Work out the finished part from the listing and answer in its coordinate system (mm). A direction names the side the tool comes from. Coordinates: 2 decimals unless noted, no trailing zeros. Order: outer loops, then holes, each group sorted by start corner. A loop starts at its lowest first (then second) coordinate and runs counter-clockwise, first axis right, second up.
```python
from build123d import *

# Parameters (mm, degrees)
BOSS_EXTRUDE1_DEPTH            = 5
FILLET1_R                      = 5
M3X0_5_TAPPED_HOLE1_AT_2_COUNT = 2
M3X0_5_TAPPED_HOLE1_AT_2_PITCH = 10
M2_5X0_45_TAPPED_HOLE2_D       = 2.05
CUT_EXTRUDE1_DEPTH             = 5
FILLET2_R                      = 3
M2_5X0_45_TAPPED_HOLE1_D       = 2.05


with BuildPart() as part:
    # Sketch1 → Boss-Extrude1 (new body)
    with BuildSketch(Plane(origin=(0, 0, 0), x_dir=(1, 0, 0), z_dir=(0, 1, 0))):
        with BuildLine():
            Line((-20.784609691, 33), (20.784609691, 33))
            ThreePointArc((20.784609691, 33), (39, 0), (20.784609691, -33))
            Line((20.784609691, -33), (-20.784609691, -33))
            ThreePointArc((-20.784609691, -33), (-39, 0), (-20.784609691, 33))
        make_face()
    extrude(amount=BOSS_EXTRUDE1_DEPTH)

    # Fillet1
    fillet1_edges = [part.edges().sort_by_distance(p)[0] for p in [
        (-20.784609691, 2.5, -33),
        (20.784609691, 2.5, -33),
        (20.784609691, 2.5, 33),
        (-20.784609691, 2.5, 33),
    ]]
    fillet(fillet1_edges, radius=FILLET1_R)

    # Sketch3 → M3x0.5 Tapped Hole1 (revolve, cut)
    with BuildSketch(Plane(origin=(-5, 2.5, 33), x_dir=(0, -1, 0), z_dir=(1, 0, 0))):
        Polygon((0, 0), (0, 8.251075774), (1.25, 7.5), (1.25, 0), align=None)
    m3x0_5_tapped_hole1 = revolve(axis=Axis((-5, 2.5, 39.35), (0, 0, -1)), mode=Mode.SUBTRACT)

    # M3x0.5 Tapped Hole1 at 2: M3x0.5 Tapped Hole1 ×2
    with Locations(*[(i * M3X0_5_TAPPED_HOLE1_AT_2_PITCH, 0, 0) for i in range(1, M3X0_5_TAPPED_HOLE1_AT_2_COUNT)]):
        add(m3x0_5_tapped_hole1, mode=Mode.SUBTRACT)

    # Mirror1: M3x0.5 Tapped Hole1 across plane
    add(m3x0_5_tapped_hole1.mirror(Plane.XY), mode=Mode.SUBTRACT)

    # Mirror1 copy 1 sketch → Mirror1 copy 1 (revolve, cut)
    with BuildSketch(Plane(origin=(5, 2.5, -33), x_dir=(0, -1, 0), z_dir=(1, 0, 0))):
        Polygon((0, 0), (0, -8.251075774), (1.25, -7.5), (1.25, 0), align=None)
    revolve(axis=Axis((5, 2.5, -39.35), (0, 0, -1)), mode=Mode.SUBTRACT)

    # M2.5x0.45 Tapped Hole2 (through all)
    with Locations(Plane(origin=(0, 0, 0), x_dir=(-1, 0, 0), z_dir=(0, -1, 0))):
        with Locations((12.5, -5), (-12.5, -5), (0, 3)):
            Hole(M2_5X0_45_TAPPED_HOLE2_D / 2)

    # Sketch6 → Cut-Extrude1 (cut)
    with BuildSketch(Plane.XZ):
        with BuildLine():
            Line((-31.749015733, 9), (31.749015733, 9))
            ThreePointArc((31.749015733, 9), (26.910919894, 19.099800796), (18.973665961, 27))
            Line((18.973665961, 27), (-18.973665961, 27))
            ThreePointArc((-18.973665961, 27), (-26.910919894, 19.099800796), (-31.749015733, 9))
        make_face()
        with BuildLine():
            Line((32.984845005, 1), (10.5, 1))
            Line((10.5, 1), (2.5, -7))
            Line((2.5, -7), (-2.5, -7))
            Line((-2.5, -7), (-10.5, 1))
            Line((-10.5, 1), (-32.984845005, 1))
            ThreePointArc((-32.984845005, 1), (-29.511382812, -14.767473872), (-18.973665961, -27))
            Line((-18.973665961, -27), (18.973665961, -27))
            ThreePointArc((18.973665961, -27), (29.511382812, -14.767473872), (32.984845005, 1))
        make_face()
    extrude(amount=-CUT_EXTRUDE1_DEPTH, mode=Mode.SUBTRACT)

    # Fillet2
    fillet2_edges = [part.edges().sort_by_distance(p)[0] for p in [
        (10.5, 2.5, 1),
        (2.5, 2.5, -7),
        (-2.5, 2.5, -7),
        (-10.5, 2.5, 1),
        (-32.984845005, 2.5, 1),
        (-18.973665961, 2.5, -27),
        (32.984845005, 2.5, 1),
        (-18.973665961, 2.5, 27),
        (31.749015733, 2.5, 9),
        (18.973665961, 2.5, 27),
        (-31.749015733, 2.5, 9),
        (18.973665961, 2.5, -27),
    ]]
    fillet(fillet2_edges, radius=FILLET2_R)

    # M2.5x0.45 Tapped Hole1 (through all)
    with Locations(Plane(origin=(0, 0, 0), x_dir=(-1, 0, 0), z_dir=(0, -1, 0))):
        with Locations((-21.15, -28.5), (21.15, -28.5), (30.3, 18.5), (-30.3, 18.5), (-35.15, -5), (35.15, -5)):
            Hole(M2_5X0_45_TAPPED_HOLE1_D / 2)


solid = part.part
```
1. The mould has two halves that part along X. Classify faces 1 (the cylindrical face through (29.98, 2.54, 10.32)), 2 (the cylindrical face through (20.75, 2.54, -32.78)), 3 (the flat face through (0, 2, -33)): released by +X, released by -X, zero draft, split by the parting line, or undercut.
2. The part is cut by section C-C (z = 28.5). Determine the outline of the cut face in (x, y) (3 decimals).
3. For faces 4 (the cylindrical face through (38.996, 2.465, -0.528)), 5 (the flat face through (-21, 2, 1)), 6 (the cylindrical face through (6.109, 1.923, 30.042)), 7 (the cylindrical face through (-3.891, 1.923, -30.042)), determine the directions among +Z, -Z, +X, -X, +Y, -Y from which every point of the face is accessible in a straight line to the end or side of a thin tool.
4. Flat-ended cylindrical pins translate along their axes: pin 1 (3 mm diameter, centred on y = 1, z = -19.5, fed in from +X); pin 2 (1.6 mm diameter, centred on x = -21.15, z = 28.5, fed in from +Y); pin 3 (1.5 mm diameter, centred on x = -21.5, y = 2, fed in from -Z). Find the tip coordinate at first contact, or state that the pin passes through.
5. The part is cut by section A-A (x = 5). Determine the outline of the cut face in (y, z), plus the area to 3 significant figures.
6. Consider probe 1 along X at (y, z) = (2.05, -18.5) (3 decimals); probe 2 along Y at (x, z) = (5, -28.35); probe 3 along Z at (x, y) = (19, 1.75). Determine where each line is inside the solid, lowest interval first.
7. The part is cut by section B-B (z = 20). Determine the outline of the cut face in (x, y), plus the area to 3 significant figures.
8. The part is cut by section D-D (x = -21.15). Determine the outline of the cut face in (y, z) (3 decimals).
Worked out:
1. face 1: undercut
1. face 2: released by +X
1. face 3: zero draft
2. outline: (-26.622, 0) - (-22.175, 0) - (-22.175, 5) - (-26.622, 5) - close; (-20.125, 0) - (20.125, 0) - (20.125, 5) - (-20.125, 5) - close; (22.175, 0) - (26.622, 0) - (26.622, 5) - (22.175, 5) - close; hole circle Ø2.5 at (-5, 2.5); hole circle Ø2.5 at (5, 2.5)
3. face 4: +X, +Y, -Y
3. face 5: +Y, -Y
3. face 6: +Z
3. face 7: -Z
4. pin 1: stops at x = 34.6
4. pin 2: passes through
4. pin 3: stops at z = -32.78
5. outline: (0, -33) - (1.25, -33) - (1.25, -27) - (0, -27) - close; (0, -4.5) - (5, -4.5) - (5, 9) - (0, 9) - close; (0, 27) - (1.25, 27) - (1.25, 33) - (0, 33) - close; (3.75, -33) - (5, -33) - (5, -27) - (3.75, -27) - close; (3.75, 27) - (5, 27) - (5, 33) - (3.75, 33) - close
5. area: 97.5 mm2
6. probe 1: x = -34.333 to -31.325, -29.275 to -27.327, 27.327 to 29.275, 31.325 to 34.333
6. probe 2: y = 0 to 1.25, 3.75 to 5
6. probe 3: z = -33 to -26.83, 1 to 9, 26.83 to 33
7. outline: (-33.48, 0) - (-26.25, 0) - (-26.25, 5) - (-33.48, 5) - close; (26.25, 0) - (33.48, 0) - (33.48, 5) - (26.25, 5) - close
7. area: 72.3 mm2
8. outline: (0, -32.64) - (5, -32.64) - (5, -25.331) - (0, -25.331) - close; (0, 1) - (5, 1) - (5, 9) - (0, 9) - close; (0, 25.331) - (5, 25.331) - (5, 27.475) - (0, 27.475) - close; (0, 29.525) - (5, 29.525) - (5, 32.64) - (0, 32.64) - close
